```python
from build123d import *

# Parameters (mm, degrees)
F0_R     = 11.5
F1_DEPTH = 2
F2_R     = 11.5
F3_DEPTH = 3
F4_R     = 8.5
F5_DEPTH = 3


with BuildPart() as f1:
    # F0 (on Top) → F1 (new body)
    with BuildSketch(Plane.XY):
        Circle(F0_R)
    extrude(amount=-F1_DEPTH)

    # F2 (on face) → F3 (join)
    with BuildSketch(Plane.XY):
        Circle(F2_R)
    extrude(amount=F3_DEPTH)

    # F4 (on face) → F5 (cut)
    with BuildSketch(Plane.XY.offset(3)):
        Circle(F4_R)
    extrude(amount=-F5_DEPTH, mode=Mode.SUBTRACT)


solid = f1.part
```
The model under review builds one solid part; all positions refer to its coordinate system, in mm. A direction names the side the tool comes from. Round coordinates to 2 decimals unless told otherwise and drop trailing zeros. Order: outer loops, then holes, each group sorted by start corner. A loop starts at its lowest first (then second) coordinate and runs counter-clockwise, first axis right, second up.
(1) Take a section at A-A, the plane x = 0. State the section outline as (y, z) points, plus the area to 3 significant figures.
Working result:
outline: (-11.5, -2) - (11.5, -2) - (11.5, 3) - (8.5, 3) - (8.5, 0) - (-8.5, 0) - (-8.5, 3) - (-11.5, 3) - close
area: 64.0 mm2
(2) Wall thickness on L1, parallel to Y at x = 0, z = 2.05; L2, parallel to Z at x = 2.5, y = 0.75; L3, parallel to Y at x = 2, z = 0.5: over which ranges is each line inside the solid? List them lowest first.
Working result:
L1: y = -11.5 to -8.5, 8.5 to 11.5
L2: z = -2 to 0
L3: y = -11.32 to -8.26, 8.26 to 11.32
(3) Mouldability with a two-part tool opening along Y and no side actions: class faces 1 (the face through (4.57, 7.167, 1.521)), 2 (the face through (0, 0, -2)) as released by +Y, released by -Y, zero draft, split by the parting line, or undercut.
Working result:
face 1: undercut
face 2: zero draft
(4) Take a section at D-D, the plane x = 10. State the section outline as (y, z) points, plus the area to 3 significant figures.
Working result:
outline: (-5.68, -2) - (5.68, -2) - (5.68, 3) - (-5.68, 3) - close
area: 56.8 mm2
(5) For P1, Ø13.5, axis at x = 0, y = 0, coming from the +Z side; P2, Ø1.5, axis at y = 3.5, z = 1, coming from the +X side; P3, Ø3, axis at x = -2.5, z = -1, coming from the -Y side, all flat-tipped, find the tip position at first contact; note any pin that passes through.
Working result:
P1: stops at z = 0
P2: stops at x = 11.17
P3: stops at y = -11.46
(6) Take a section at C-C, the plane z = 0.6. State the section outline as (x, y) points.
Working result:
outline: circle Ø23 at (0, 0); hole circle Ø17 at (0, 0)
(7) Tool access review of faces 3 (the face through (0, 0, 0)), 4 (the face through (-4, -8, 3)): name each direction out of +Z, -Z, +X, -X, +Y, -Y from which nothing blocks a thin tool from reaching the whole face with its end or side.
Working result:
face 3: +Z
face 4: +Z, +X, -X, +Y, -Y
